The drawing under review shows one solid part. Ordinate dimensions are in mm from its lowest x, y, z. A direction names the side the tool comes from. Coordinates: 2 decimals unless noted, no trailing zeros. Loops run counter-clockwise (first coordinate to the right, second up) from the corner with the lowest first, then second, coordinate; pieces in that order, holes last. Notation, with made-up numbers: M 38.25,23.5 L 62.25,23.5 A14 cw 62.25,46.5 Z; hole C 16.25,21.25 d2. An arc over 180 degrees is marked long. Put each result on its own line as item: value.
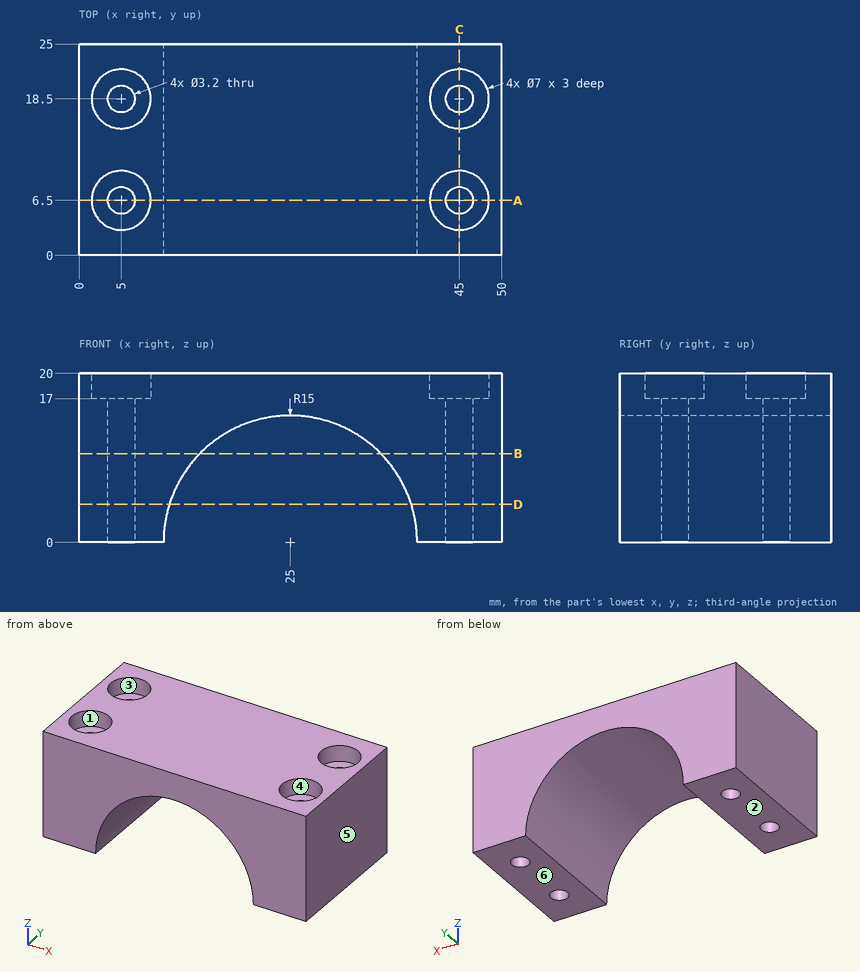
(1) Add section C-C (x = 45). Write out the cut boundary in (y, z), plus the area to 3 significant figures.
Determined:
outline: M 0,0 L 4.9,0 L 4.9,17 L 3,17 L 3,20 L 0,20 Z; M 8.1,0 L 16.9,0 L 16.9,17 L 15,17 L 15,20 L 10,20 L 10,17 L 8.1,17 Z; M 20.1,0 L 25,0 L 25,20 L 22,20 L 22,17 L 20.1,17 Z
area: 349 mm^2
(2) Tool access review of the marked faces 1 and 2: name each direction out of +Z, -Z, +X, -X, +Y, -Y from which nothing blocks a thin tool from reaching the whole face with its end or side.
Determined:
face 1: +Z
face 2: -Z, +X, -X, +Y, -Y
(3) Draft analysis for pull direction X (two halves, no side actions). For the marked faces 3, 4, 5 and 6, state which applies: +X half, -X half, draft (parallel to the pull), parting line (faces both ways), or undercut.
Determined:
face 3: undercut
face 4: undercut
face 5: +X half
face 6: draft
(4) Add section D-D (z = 4.5). Write out the cut boundary in (x, y).
Determined:
outline: M 0,0 L 10.69,0 L 10.69,25 L 0,25 Z; M 39.31,0 L 50,0 L 50,25 L 39.31,25 Z; hole C 5,6.5 d3.2; hole C 5,18.5 d3.2; hole C 45,6.5 d3.2; hole C 45,18.5 d3.2
(5) For pin 1 (8 mm diameter, centred on x = 27.5, y = 13.5, fed in from -Z); pin 2 (4 mm diameter, centred on x = 5, y = 6.5, fed in from +Z); pin 3 (3 mm diameter, centred on x = 5, y = 18.5, fed in from -Z); pin 4 (1 mm diameter, centred on x = 23, y = 12, fed in from -Z), all flat-tipped, find the tip position at first contact; note any pin that passes through.
Determined:
pin 1: stops at z = 13.52
pin 2: stops at z = 17
pin 3: passes through
pin 4: stops at z = 14.79
(6) Add section B-B (z = 10.5). Write out the cut boundary in (x, y), plus the area to 3 significant figures.
Determined:
outline: M 0,0 L 14.29,0 L 14.29,25 L 0,25 Z; M 35.71,0 L 50,0 L 50,25 L 35.71,25 Z; hole C 5,6.5 d3.2; hole C 5,18.5 d3.2; hole C 45,6.5 d3.2; hole C 45,18.5 d3.2
area: 682 mm^2
(7) Add section A-A (y = 6.5). Write out the cut boundary in (x, z), plus the area to 3 significant figures.
Determined:
outline: M 0,0 L 3.4,0 L 3.4,17 L 1.5,17 L 1.5,20 L 0,20 Z; M 6.6,0 L 10,0 A15 cw 40,0 L 43.4,0 L 43.4,17 L 41.5,17 L 41.5,20 L 8.5,20 L 8.5,17 L 6.6,17 Z; M 46.6,0 L 50,0 L 50,20 L 48.5,20 L 48.5,17 L 46.6,17 Z
area: 496 mm^2
(8) Wall thickness on line 1 along Y through (x, z) = (5, 18.65); line 2 along Y through (x, z) = (5, 12); line 3 along X through (y, z) = (19, 7): over which ranges is each line inside the solid? List them lowest first. Write a range as [from, to].
Determined:
line 1: y = [0, 3], [10, 15], [22, 25]
line 2: y = [0, 4.9], [8.1, 16.9], [20.1, 25]
line 3: x = [0, 3.48], [6.52, 11.73], [38.27, 43.48], [46.52, 50]
